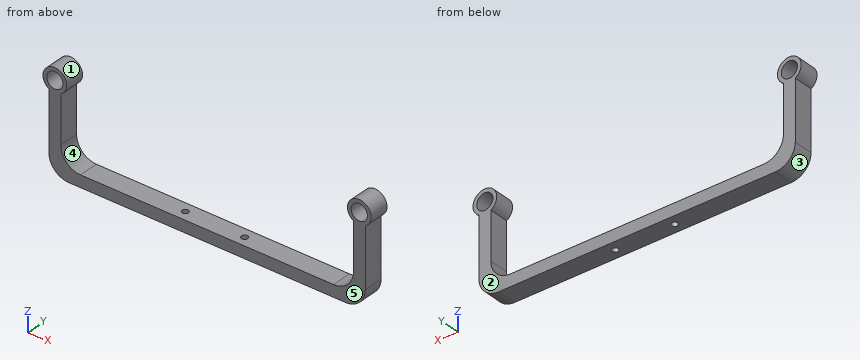
from build123d import *

# Parameters (mm, degrees)
SKETCH_1_R          = 4.1
EXTRUDE_1_DEPTH     = 10
SKETCH_3_R          = 1.6
CUT_EXTRUDE_1_DEPTH = 52.196152423
FILLET_1_R          = 10


with BuildPart() as part:
    # Эскиз1 → Бобышка-Вытянуть1 (new body)
    with BuildSketch(Plane(origin=(0, 0, 0), x_dir=(1, 0, 0), z_dir=(0, 1, 0))):
        with BuildLine():
            Line((-63.596685083, 9.903314917), (96.403314917, 9.903314917))
            Line((96.403314917, 9.903314917), (96.403314917, -30.096685083))
            ThreePointArc((96.403314917, -30.096685083), (93.403314917, -41.292837506), (90.403314917, -30.096685083))
            Line((90.403314917, -30.096685083), (90.403314917, 3.903314917))
            Line((90.403314917, 3.903314917), (-57.596685083, 3.903314917))
            Line((-57.596685083, 3.903314917), (-57.596685083, -30.096685083))
            ThreePointArc((-57.596685083, -30.096685083), (-60.596685083, -41.292837506), (-63.596685083, -30.096685083))
            Line((-63.596685083, -30.096685083), (-63.596685083, 9.903314917))
        make_face()
        with Locations((-60.596685083, -35.292837506)):
            Circle(SKETCH_1_R, mode=Mode.SUBTRACT)
        with Locations((93.403314917, -35.292837506)):
            Circle(SKETCH_1_R, mode=Mode.SUBTRACT)
    extrude(amount=EXTRUDE_1_DEPTH)

    # Эскиз3 → Вырез-Вытянуть1 (cut, through all)
    with BuildSketch(Plane(origin=(0, 0, -9.903314917), x_dir=(-1, 0, 0), z_dir=(0, 0, -1))):
        with Locations((-1.403314917, 5)):
            Circle(SKETCH_3_R)
        with Locations((-31.403314917, 5)):
            Circle(SKETCH_3_R)
    extrude(amount=-CUT_EXTRUDE_1_DEPTH, mode=Mode.SUBTRACT)

    # Скругление1
    fillet_1_edges = [part.edges().sort_by_distance(p)[0] for p in [
        (-63.596685083, 5, -9.903314917),
        (96.403314917, 5, -9.903314917),
        (90.403314917, 5, -3.903314917),
        (-57.596685083, 5, -3.903314917),
    ]]
    fillet(fillet_1_edges, radius=FILLET_1_R)


solid = part.part
Build history of the part. All positions in model axes, mm. Face numbers are marked on the shaded views. A direction names the side the tool comes from. Coordinates: 2 decimals unless noted, no trailing zeros. Write each loop counter-clockwise with the first axis right and the second up, starting at its lowest first coordinate (ties: lowest second). Pieces come first, ordered by that corner, then holes.
(1) Drill centre lines: line 1 (X direction, y = 5.5, z = 35); line 2 (X direction, y = 6, z = 26); line 3 (X direction, y = 9.5, z = 33). Where is each one in solid material? Low to high.
(2) Cut at B-B on y = 5. List the corners of the cut face in (x, z).
(3) Cut at C-C on z = 33. List the corners of the cut face in (x, y), and give its area (3 significant figures).
(4) 3-axis set-ups, long thin cutter, end or side, ignore diameter. For the marked faces 4 and 5: which of +Z, -Z, +X, -X, +Y, -Y reach the whole face in a straight line?
(5) Cut at A-A on z = 26.5. List the corners of the cut face in (x, y).
(6) Mould opens along Z. For the marked faces 1, 2 and 3 say: pulls with the +Z half, pulls with the -Z half, needs draft (parallel to the pull), parting line crosses it, or undercut.
(7) Cut at D-D on x = 52.5. List the corners of the cut face in (y, z).
(8) Pin check, flat tips, straight feed: pin 1 Ø2 at (y, z) = (7, 27) entering from -X; pin 2 Ø2 at (y, z) = (1.5, 10.5) entering from +X; pin 3 Ø3.5 at (x, y) = (31.4, 5) entering from +Z; pin 4 Ø13 at (x, z) = (93.4, 35.29) entering from +Y. Stop position of each tip, or through.
Working result:
1. line 1: x = -66.59 to -64.69, -56.51 to -54.6, 87.41 to 89.31, 97.49 to 99.4
1. line 2: x = -63.6 to -57.6, 90.4 to 96.4
1. line 3: x = -66.14 to -64, -57.2 to -55.05, 87.86 to 90, 96.8 to 98.95
2. outline: (-63.6, 0.1) arc R10 ccw to (-53.6, -9.9) - (-0.2, -9.9) - (-0.2, -3.9) - (-47.6, -3.9) arc R10 cw to (-57.6, 6.1) - (-57.6, 30.1) arc R6 ccw (long way) to (-63.6, 30.1) - close; (3, -9.9) - (29.8, -9.9) - (29.8, -3.9) - (3, -3.9) - close; (33, -9.9) - (86.4, -9.9) arc R10 ccw to (96.4, 0.1) - (96.4, 30.1) arc R6 ccw (long way) to (90.4, 30.1) - (90.4, 6.1) arc R10 cw to (80.4, -3.9) - (33, -3.9) - close; hole circle Ø8.2 at (-60.6, 35.29); hole circle Ø8.2 at (93.4, 35.29)
3. outline: (-66.14, 0) - (-64, 0) - (-64, 10) - (-66.14, 10) - close; (-57.2, 0) - (-55.05, 0) - (-55.05, 10) - (-57.2, 10) - close; (87.86, 0) - (90, 0) - (90, 10) - (87.86, 10) - close; (96.8, 0) - (98.95, 0) - (98.95, 10) - (96.8, 10) - close
3. area: 85.8 mm2
4. face 4: +Y, -Y
4. face 5: +Z, -Z, +X, -X, -Y
5. outline: (-63.6, 0) - (-57.6, 0) - (-57.6, 10) - (-63.6, 10) - close; (90.4, 0) - (96.4, 0) - (96.4, 10) - (90.4, 10) - close
6. face 1: undercut
6. face 2: needs draft
6. face 3: pulls with the -Z half
7. outline: (0, -9.9) - (10, -9.9) - (10, -3.9) - (0, -3.9) - close
8. pin 1: stops at x = -63.6
8. pin 2: stops at x = 96.4
8. pin 3: stops at z = -3.9
8. pin 4: stops at y = 10
